Here's how the part is built. I have some questions about the finished solid (model axes, mm). A direction names the side the tool comes from. Round coordinates to 2 decimals unless told otherwise and drop trailing zeros. Loops run counter-clockwise (first coordinate to the right, second up) from the corner with the lowest first, then second, coordinate; pieces in that order, holes last. Notation, with made-up numbers: M -32,11.5 L 24,11.5 A29 cw 24,46.5 Z; hole C -34,-37.75 d3. An arc over 180 degrees is marked long. Use a Markdown table: item, result.
Autodesk Inventor part; units mm, degrees
ref_plane "YZ Plane" through (0, 0, 0) normal (1, 0, 0) x (0, 1, 0)
ref_plane "XZ Plane" through (0, 0, 0) normal (0, 1, 0) x (-1, 0, 0)
ref_plane "XY Plane" through (0, 0, 0) normal (0, 0, 1) x (1, 0, 0)
sketch "Sketch1" plane through (0, 0, 0) normal (1, 0, 0) x (0, 1, 0)
  line L0 (0, 0) -> (250, 0)
  line L1 (250, 0) -> (250, 270)
  line L2 (250, 270) -> (0, 270)
  line L3 (0, 270) -> (0, 0)
  dimension "d0" = 250
  dimension "d1" = 270
extrude "Extrusion1" add sketch "Sketch1" along normal blind 250
shell "Shell1" thickness 2 removed faces 1 at (166.6667, 166.6667, 270)
sketch "Sketch2" plane through (0, 250, 270) normal (0, 1, 0) x (1, 0, 0)
  point P0 (0, 270)
sketch "Sketch3" plane through (2, 248, 2) normal (0, -1, 0) x (1, 0, 0)
  line L0 (0, 268) -> (246, 268)
  line L1 (0, 268) -> (246, 268)
  line L2 (246, 268) -> (246, 266)
  line L3 (246, 266) -> (0, 266)
  line L4 (0, 266) -> (0, 268)
  point P0 (-2, -2)
  dimension "d5" = 246
  dimension "d6" = 2
extrude "Extrusion2" add sketch "Sketch3" along normal blind 246
properties part number "Caja grande"
1. For pin 1 Ø1 at (x, y) = (215.5, 95.5) entering from -Z, with a flat end and sliding along its axis, tell me the tip position at first contact or that it passes through.
Answer sheet:
| item | result |
|---|---|
| pin 1 | z = 0 |
2. We'd pull the mould along Y, two halves only. Please class faces 3 (the face through (123, 127, 270)), 4 (the face through (123, 123, 2)), 5 (the face through (123, 0, 137)): +Y half, -Y half, draft (parallel to the pull), parting line (faces both ways), or undercut.
Answer sheet:
| item | result |
|---|---|
| face 3 | draft |
| face 4 | undercut |
| face 5 | -Y half |
3. I need wall thicknesses on probe 1 along X at (y, z) = (154, 247); probe 2 along Z at (x, y) = (186, 180.5). Which ranges of each line are inside material? Lowest first, please. Write a range as from..to.
Answer sheet:
| item | result |
|---|---|
| probe 1 | 0..2, 248..250 |
| probe 2 | 0..2, 268..270 |
4. Imagine slicing it at A-A, the plane x = 201. Write out the boundary of the cut face in (y, z).
Answer sheet:
| item | result |
|---|---|
| outline | M 0,0 L 250,0 L 250,270 L 0,270 Z; hole M 2,2 L 248,2 L 248,268 L 2,268 Z |
5. Which directions (+Z, -Z, +X, -X, +Y, -Y) give clear straight access to the entire face, cutting with the end or side of a thin tool? Please do faces 1 (the face through (127, 127, 268)), 2 (the face through (0, 123, 137)).
Answer sheet:
| item | result |
|---|---|
| face 1 | none |
| face 2 | +Z, -Z, -X, +Y, -Y |
